Build history of the part. All positions in model axes, mm. Face numbers are marked on the shaded views. Give positions to 0.01 mm unless a question says otherwise; leave off trailing zeros. Loops run counter-clockwise (first coordinate to the right, second up) from the corner with the lowest first, then second, coordinate; pieces in that order, holes last. Notation, with made-up numbers: M 3.5,25.25 L 59.5,25.25 A16 cw 59.5,31.25 Z; hole C 61.5,-13 d10. An arc over 180 degrees is marked long. Put each result on its own line as item: value.
Autodesk Inventor part; units mm, degrees
ref_plane "inner_ring_XY" through (0, 0, 0) normal (0, 0, 1) x (1, 0, 0)
ref_plane "inner_ring_YZ" through (0, 0, 0) normal (1, 0, 0) x (0, 1, 0)
ref_plane "inner_ring_ZX" through (0, 0, 0) normal (0, 1, 0) x (0, 0, 1)
sketch "Sketch_1" plane through (0, 0, 0) normal (0, 0, 1) x (1, 0, 0)
  line L0 (16, 0) -> (0, 0)
  line L1 (0, 32.6773) -> (0, 30)
  line L2 (0, 30) -> (16, 30)
  arc A0 (16, 30) -> (17, 31) centre (16, 31) ccw
  line L3 (17, 31) -> (17, 36.65)
  line L4 (17, 36.65) -> (16.75, 36.9)
  line L5 (16.75, 36.9) -> (14.0638, 36.9)
  line L6 (14.0638, 36.9) -> (14.4927, 34.9577)
  line L7 (14.4927, 34.9577) -> (1.8039, 32.3617)
  line L8 (1.8039, 32.3617) -> (1.6171, 33.2081)
  line L9 (1.6171, 33.2081) -> (0.1959, 32.9174)
  line L10 (0.1959, 32.9174) -> (0, 32.6773)
revolve "Revolution1" add sketch "Sketch_1" angle 360 about axis through (16, 0, 0) along (1, 0, 0)
ref_plane "inner_ring_XY" through (0, 0, 0) normal (0, 0, 1) x (1, 0, 0)
ref_plane "inner_ring_YZ" through (0, 0, 0) normal (1, 0, 0) x (0, 1, 0)
ref_plane "inner_ring_ZX" through (0, 0, 0) normal (0, 1, 0) x (0, 0, 1)
properties part number "32912_ir"
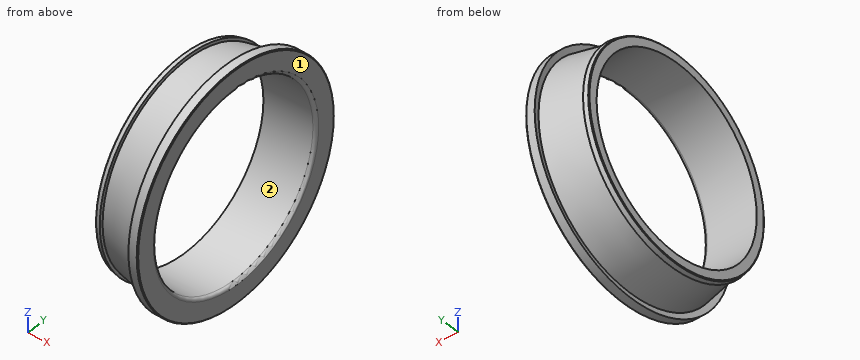
Q1. Slice it at C-C (x = 5). List the corners of the cut face in (y, z), and give its area (3 significant figures).
Here are the results:
outline: C 0,0 d66.03; hole C 0,0 d60
area: 597 mm²
Q2. Slice it at A-A (y = 0). List the corners of the cut face in (x, z).
Here are the results:
outline: M 0,-32.68 L 0.2,-32.92 L 1.62,-33.21 L 1.8,-32.36 L 14.49,-34.96 L 14.06,-36.9 L 16.75,-36.9 L 17,-36.65 L 17,-31 A1 ccw 16,-30 L 0,-30 Z; M 0,30 L 16,30 A1 ccw 17,31 L 17,36.65 L 16.75,36.9 L 14.06,36.9 L 14.49,34.96 L 1.8,32.36 L 1.62,33.21 L 0.2,32.92 L 0,32.68 Z
Q3. Mould opens along Y. For the marked faces 1 and 2 say: pulls with the +Y half, pulls with the -Y half, needs draft (parallel to the pull), parting line crosses it, or undercut.
Here are the results:
face 1: needs draft
face 2: undercut
Q4. Slice it at D-D (x = 12.75). List the corners of the cut face in (y, z).
Here are the results:
outline: C 0,0 d69.2; hole C 0,0 d60
Q5. Probe line 1 (Z direction, x = 5, y = 0); line 2 (Z direction, x = 6.75, y = 17); line 3 (Y direction, x = 16.25, z = -12). List the from-to ranges inside material, lowest first. Write a range as from..to.
Here are the results:
line 1: -33.02..-30, 30..33.02
line 2: -28.72..-24.72, 24.72..28.72
line 3: -34.89..-27.53, 27.53..34.89
Q6. Drop flat-ended pins along their axis: pin 1 Ø3 at (x, y) = (10, 10.5) entering from +Z; pin 2 Ø3 at (x, y) = (4, -5) entering from +Z; pin 3 Ø2 at (x, y) = (5, 17) entering from -Z. Give the stop position or say it passes through.
Here are the results:
pin 1: z = 32.93
pin 2: z = 32.8
pin 3: z = -28.93
